Autodesk Inventor part; units mm, degrees
ref_plane "YZ Plane" through (0, 0, 0) normal (1, 0, 0) x (0, 1, 0)
ref_plane "XZ Plane" through (0, 0, 0) normal (0, 1, 0) x (-1, 0, 0)
ref_plane "XY Plane" through (0, 0, 0) normal (0, 0, 1) x (1, 0, 0)
sketch "Sketch1" plane through (0, 0, 0) normal (0, 1, 0) x (-1, 0, 0)
  line L0 (0, 0) -> (0, -355.998) construction
  line L1 (5, 0) -> (5, -355.998)
  line L2 (-5, -355.998) -> (-5, 0)
  arc A0 (5, 0) -> (-5, 0) centre (0, 0) ccw
  arc A1 (-5, -355.998) -> (5, -355.998) centre (0, -355.998) ccw
  circle A2 centre (0, 0) radius 1.65
  circle A3 centre (0, -355.998) radius 1.65
  circle A4 centre (0, -57.376) radius 1.65
  point P0 (0, -177.999)
  dimension "d0" = 3.3
  dimension "d1" = 3.3
  dimension "d2" = 10
  dimension "d3" = 355.998
  dimension "d14" = 3.3
  dimension "d15" = 57.376
extrude "Extrusion1" add sketch "Sketch1" along normal blind 3
sketch "Sketch2" plane through (0, 3, 0) normal (0, 1, 0) x (1, 0, 0)
  line L0 (-26.2185, 378.6248) -> (37.2853, 378.6248)
  line L1 (37.2853, 378.6248) -> (37.2853, 176.2061)
  line L2 (37.2853, 176.2061) -> (-26.2185, 176.2061)
  line L3 (-26.2185, 176.2061) -> (-26.2185, 378.6248)
  line L4 (-95.1798, 405.4155) -> (74.9908, 405.4155)
  line L5 (74.9908, 405.4155) -> (74.9908, -44.073)
  line L6 (74.9908, -44.073) -> (-95.1798, -44.073)
  line L7 (-95.1798, -44.073) -> (-95.1798, 405.4155)
  point P0 (0, 0)
extrude "Extrusion2" cut sketch "Sketch2" against normal blind 10 contours L0 L1 L2 L3
properties part number "Part_10_p1"
Part model, mm, in its own coordinate system. Round coordinates to 2 decimals unless told otherwise and drop trailing zeros. Loops run counter-clockwise (first coordinate to the right, second up) from the corner with the lowest first, then second, coordinate; pieces in that order, holes last. Notation, with made-up numbers: (58, 78) -> (114, 78) arc R15 ccw to (114, 93) -> close; hole circle Ø8 at (36.5, 65.25). An arc over 180 degrees is marked (long way). Use CSV: the item, a comma, the result in double quotes. Start each with the question number.
1) Wall check: L1, parallel to Z at x = 0, y = 1.15; L2, parallel to Z at x = 0.5, y = 0.9; L3, parallel to Z at x = -4, y = 0.5. Give the ranges that are in metal, low to high. Write a range as [from, to].
2) Cut at A-A, the plane x = 0. Write the cut outline in (y, z), plus the area to 3 significant figures.
3) Pull direction Z, two halves, no side cores. Call faces 1 (the cylindrical face through (1.216, 1.479, -1.115)), 2 (the flat face through (-5, 1, -87)), 3 (the cylindrical face through (-0.887, 1.479, -58.767)), 4 (the flat face through (0, 2, -176.206)): +Z half, -Z half, draft (parallel to the pull), parting line (faces both ways), or undercut.
4) Cut at B-B, the plane y = 2.1. Write the cut outline in (x, z).
Determined:
1,L1,"z = [-176.21, -59.03], [-55.73, -1.65], [1.65, 5]"
1,L2,"z = [-176.21, -58.95], [-55.8, -1.57], [1.57, 4.97]"
1,L3,"z = [-176.21, 3]"
2,outline,"(0, -176.21) -> (3, -176.21) -> (3, -59.03) -> (0, -59.03) -> close; (0, -55.73) -> (3, -55.73) -> (3, -1.65) -> (0, -1.65) -> close; (0, 1.65) -> (3, 1.65) -> (3, 5) -> (0, 5) -> close"
2,area,"524 mm2"
3,face 1,"undercut"
3,face 2,"draft"
3,face 3,"undercut"
3,face 4,"-Z half"
4,outline,"(-5, -176.21) -> (5, -176.21) -> (5, 0) arc R5 ccw to (-5, 0) -> close; hole circle Ø3.3 at (0, -57.38); hole circle Ø3.3 at (0, 0)"
